Source: CAD feature listing. Evaluate the final solid. Frame: model axes, mm. A direction names the side the tool comes from. Coordinates: 2 decimals unless noted, no trailing zeros. Order: outer loops, then holes, each group sorted by start corner. A loop starts at its lowest first (then second) coordinate and runs counter-clockwise, first axis right, second up. Notation, with made-up numbers: (66.5, 69) -> (116.5, 69) arc R14 ccw to (116.5, 86) -> close; hole circle Ø9 at (-18.75, -4). An arc over 180 degrees is marked (long way). Put each result on its own line as item: value.
Autodesk Inventor part; units mm, degrees
ref_plane "YZ Plane" through (0, 0, 0) normal (1, 0, 0) x (0, 1, 0)
ref_plane "XZ Plane" through (0, 0, 0) normal (0, 1, 0) x (-1, 0, 0)
ref_plane "XY Plane" through (0, 0, 0) normal (0, 0, 1) x (1, 0, 0)
sketch "Sketch1" plane through (0, 0, 0) normal (0, 0, 1) x (1, 0, 0)
  circle A0 centre (0, 0) radius 25
  circle A1 centre (0, 0) radius 17.5
  dimension "d0" = 35
  dimension "d1" = 50
extrude "Extrusion1" add sketch "Sketch1" along normal mid plane 50 contours A1
extrude "Extrusion2" add sketch "Sketch1" along normal mid plane 70
chamfer "Chamfer1" distance 5 angle 45 1 edges at (-17.5, 0, 35)
chamfer "Chamfer2" distance 1 angle 45 1 edges at (-25, 0, 35)
chamfer "Chamfer3" distance 3 angle 45 2 edges at (-17.5, 0, -25) (-17.5, 0, -35)
properties part number "LENS"
1. First-contact query: pin 1 (12 mm diameter, centred on x = -6, z = 24.5, fed in from -Y); pin 2 (3 mm diameter, centred on x = -11, y = 0.5, fed in from +Z); pin 3 (4 mm diameter, centred on x = 1, z = 11, fed in from +Y). Flat tips, straight axial feed; report the tip coordinate or a pass-through.
Numbers:
pin 1: stops at y = -25
pin 2: stops at z = 25
pin 3: stops at y = 25
2. Cut plane A-A on y = 0. Output: boundary loops of the cut face in (x, z).
Numbers:
outline: (-25, -35) -> (-20.5, -35) -> (-17.5, -32) -> (-17.5, -28) -> (-14.5, -25) -> (14.5, -25) -> (17.5, -28) -> (17.5, -32) -> (20.5, -35) -> (25, -35) -> (25, 34) -> (24, 35) -> (22.5, 35) -> (17.5, 30) -> (17.5, 25) -> (-17.5, 25) -> (-17.5, 30) -> (-22.5, 35) -> (-24, 35) -> (-25, 34) -> close
3. Ray query, line 1 along Y through (x, z) = (0, 28); line 2 along Z through (x, y) = (13, 4); line 3 along X through (y, z) = (7, -8). Return the intervals inside material, ascending.
Numbers:
line 1: y = -25 to -17.5, 17.5 to 25
line 2: z = -25 to 25
line 3: x = -24 to 24
4. Pull-direction query (Y, two-part tool) for faces 4 (the conical face through (14.01, -4.41, -25.19)), 5 (the flat face through (14, -18, 35)), 6 (the cylindrical face through (-13.887, 10.648, 27.465)), 7 (the cylindrical face through (23.846, -7.509, -0.983)); classes: pulls with the +Y half, pulls with the -Y half, needs draft (parallel to the pull), parting line crosses it, or undercut.
Numbers:
face 4: undercut
face 5: needs draft
face 6: undercut
face 7: parting line crosses it
5. Cut plane C-C on z = -19. Output: boundary loops of the cut face in (x, y).
Numbers:
outline: circle Ø50 at (0, 0)
6. Set-up query: faces 1 (the flat face through (0, 0, -25)), 2 (the flat face through (0, 0, 25)), 3 (the flat face through (-3.8, 20.5, -35)). Return all of +Z, -Z, +X, -X, +Y, -Y with unobstructed straight access to the full face (end or side cutting, diameter ignored); none if empty.
Numbers:
face 1: -Z
face 2: +Z
face 3: -Z, +X, -X, +Y, -Y
